Could you check a few things on this model? Use its own coordinates, in mm. A direction names the side the tool comes from. Give positions to 0.01 mm unless a question says otherwise; leave off trailing zeros. Write each loop counter-clockwise with the first axis right and the second up, starting at its lowest first coordinate (ties: lowest second). Pieces come first, ordered by that corner, then holes. Notation, with made-up numbers: (12.5, 5.25) - (71.5, 5.25) arc R29 cw to (71.5, 42.25) - close; hole circle Ø8 at (45.5, 46). An arc over 180 degrees is marked (long way). Answer as CSV lines item,"result". Start each with the question number.
Q1. We'd pull the mould along Z, two halves only. Please class faces 3 (the face through (32, 309, -10)), 4 (the face through (25, 301, 0)), 5 (the face through (8, 0, -51)), 6 (the face through (25, 309, -100)): pulls with the +Z half, pulls with the -Z half, needs draft (parallel to the pull), parting line crosses it, or undercut.
Q2. Imagine slicing it at C-C on z = -33. List the corners of the cut face in (x, y) for me, and give its area (3 significant figures).
Q3. Imagine slicing it at A-A on x = 20. List the corners of the cut face in (y, z) for me, and give its area (3 significant figures).
Q4. Imagine slicing it at B-B on y = 180. List the corners of the cut face in (x, z) for me, and give its area (3 significant figures).
Q5. If I drill on line 1 along Z through (x, y) = (27, 176); line 2 along X through (y, z) = (462.5, -30.5); line 3 along Z through (x, y) = (11.5, 149.5), over which ranges is the centre line in solid material (lowest first)?
Q6. On a 3-axis mill with a long thin cutter (end or side, diameter ignored), from which of +Z, -Z, +X, -X, +Y, -Y can I reach the whole of each face in a straight line? I mean faces 1 (the face through (50, 301, -5)), 2 (the face through (32, 301, -90)). Say none if no direction works.
Q7. Will these pins go through, and if not, where does the flat tip stop? pin 1 Ø8 at (y, z) = (489.5, -63.5) entering from +X; pin 2 Ø2 at (x, y) = (29.5, 140) entering from +Z.
Autodesk Inventor part; units mm, degrees
ref_plane "YZ Plane" through (0, 0, 0) normal (1, 0, 0) x (0, 1, 0)
ref_plane "XZ Plane" through (0, 0, 0) normal (0, 1, 0) x (-1, 0, 0)
ref_plane "XY Plane" through (0, 0, 0) normal (0, 0, 1) x (1, 0, 0)
sketch "Sketch1" plane through (0, 0, 0) normal (1, 0, 0) x (0, 1, 0)
  line L0 (0, 0) -> (610, 0)
  line L1 (610, 0) -> (610, -100)
  line L2 (610, -100) -> (0, -100)
  line L3 (0, -100) -> (0, 0)
  dimension "d0" = 610
  dimension "d1" = 100
extrude "Extrusion1" add sketch "Sketch1" along normal blind 50
sketch "Sketch2" plane through (50, 0, 0) normal (1, 0, 0) x (0, 0, -1)
  line L0 (0, 0) -> (100, 0)
  line L1 (100, 610) -> (0, 610)
  line L2 (10, 0) -> (90, 0)
  line L3 (90, 0) -> (90, 610)
  line L4 (90, 610) -> (10, 610)
  line L5 (10, 610) -> (10, 0)
  dimension "d4" = 80
extrude "Extrusion2" cut sketch "Sketch2" against normal blind 40
fillet "Fillet1" radius 4 2 edges at (10, 305, -90) (10, 305, -10)
equation "\"BendRadius\" = Thickness"
equation "\"BendReliefWidth\" = Thickness"
equation "\"BendReliefDepth\" = 0.5 * Thickness"
equation "\"CornerReliefSize\" = 4 * Thickness"
equation "\"MinimumRemnant\" = 2 * Thickness"
equation "\"TransitionRadius\" = BendRadius"
equation "\"JacobiRadiusSize\" = BendRadius"
equation "\"GapSize\" = Thickness"
properties part number "Base3"
Conclusion:
1,face 3,"undercut"
1,face 4,"pulls with the +Z half"
1,face 5,"needs draft"
1,face 6,"pulls with the -Z half"
2,outline,"(0, 0) - (10, 0) - (10, 610) - (0, 610) - close"
2,area,"6,100 mm^2"
3,outline,"(0, -100) - (610, -100) - (610, -90) - (0, -90) - close; (0, -10) - (610, -10) - (610, 0) - (0, 0) - close"
3,area,"12,200 mm^2"
4,outline,"(0, -100) - (50, -100) - (50, -90) - (14, -90) arc R4 cw to (10, -86) - (10, -14) arc R4 cw to (14, -10) - (50, -10) - (50, 0) - (0, 0) - close"
4,area,"1,810 mm^2"
5,line 1,"-100 to -90, -10 to 0"
5,line 2,"0 to 10"
5,line 3,"-100 to -89.12, -10.88 to 0"
6,face 1,"+Z, -Z, +X, +Y, -Y"
6,face 2,"+X, +Y, -Y"
7,pin 1,"x = 10"
7,pin 2,"z = 0"
